CAD build for the part. Positions are in the model's coordinates, mm. A direction names the side the tool comes from. Give positions to 0.01 mm unless a question says otherwise; leave off trailing zeros. Loops run counter-clockwise (first coordinate to the right, second up) from the corner with the lowest first, then second, coordinate; pieces in that order, holes last. Notation, with made-up numbers: M 38.25,63.25 L 52.25,63.25 A29 cw 52.25,99.25 Z; hole C -14.5,-27 d10. An arc over 180 degrees is marked long. One line per question, with ' | ' between items.
```python
from build123d import *

# Parameters (mm, degrees)
BOSS_EXTRUDE1_DEPTH = 2
SKETCH2_R           = 3
SKETCH2_R_2         = 3.5
BOSS_EXTRUDE2_DEPTH = 3
SKETCH3_R           = 1.6
SKETCH3_R_2         = 2.1
CUT_EXTRUDE1_DEPTH  = 6


with BuildPart() as part:
    # Sketch1 → Boss-Extrude1 (new body)
    with BuildSketch(Plane.XY):
        with BuildLine():
            Line((0, 3), (6, 3))
            ThreePointArc((6, 3), (8.121320344, 3.878679656), (9, 6))
            Line((9, 6), (9, 12.5))
            ThreePointArc((9, 12.5), (9.878679656, 14.621320344), (12, 15.5))
            Line((12, 15.5), (21.823666576, 15.995555253))
            ThreePointArc((21.823666576, 15.995555253), (24.411724799, 15.036450964), (25.5, 12.5))
            Line((25.5, 12.5), (25.5, -7.5))
            ThreePointArc((25.5, -7.5), (23.339392013, -10.733578364), (19.525126266, -9.974873734))
            Line((19.525126266, -9.974873734), (12.550252532, -3))
            Line((12.550252532, -3), (0, -3))
            ThreePointArc((0, -3), (-3, 0), (0, 3))
        make_face()
    extrude(amount=BOSS_EXTRUDE1_DEPTH)

    # Sketch2 → Boss-Extrude2 (add)
    with BuildSketch(Plane.XY.offset(2)):
        Circle(SKETCH2_R)
        with Locations((12, 12.5)):
            Circle(SKETCH2_R)
        with Locations((22, 12.5)):
            Circle(SKETCH2_R_2)
        with Locations((22, -7.5)):
            Circle(SKETCH2_R_2)
    extrude(amount=BOSS_EXTRUDE2_DEPTH)

    # Sketch3 → Cut-Extrude1 (cut, through all)
    with BuildSketch(Plane.XY.offset(5)):
        Circle(SKETCH3_R)
        with Locations((12, 12.5)):
            Circle(SKETCH3_R)
        with Locations((22, 12.5)):
            Circle(SKETCH3_R_2)
        with Locations((22, -7.5)):
            Circle(SKETCH3_R_2)
    extrude(amount=-CUT_EXTRUDE1_DEPTH, mode=Mode.SUBTRACT)


solid = part.part
```
Item 1: Saw through at B-B on y = 0. Give the cut face in (x, z).
Conclusion:
outline: M -3,0 L -1.6,0 L -1.6,5 L -3,5 Z; M 1.6,0 L 25.5,0 L 25.5,2 L 3,2 L 3,5 L 1.6,5 Z
Item 2: Saw through at A-A on z = 3.8. Give the cut face in (x, y).
Conclusion:
outline: C 0,0 d6; C 12,12.5 d6; C 22,-7.5 d7; C 22,12.5 d7; hole C 0,0 d3.2; hole C 12,12.5 d3.2; hole C 22,-7.5 d4.2; hole C 22,12.5 d4.2
Item 3: 3-axis set-ups, long thin cutter, end or side, ignore diameter. For faces 1 (the flat face through (3, 3, 1)), 2 (the cylindrical face through (24.003, 13.131, 2.535)), 3 (the flat face through (16, 3, 2)), 4 (the flat face through (24, 11, 5)), 5 (the flat face through (6, -3, 1)): which of +Z, -Z, +X, -X, +Y, -Y reach the whole face in a straight line?
Conclusion:
face 1: +Z, -Z, -X, +Y | face 2: +Z, -Z | face 3: +Z | face 4: +Z, +X, -X, +Y, -Y | face 5: +Z, -Z, -X, -Y
Item 4: Mould opens along X. For faces 6 (the flat face through (9, 9, 1)), 7 (the flat face through (13, 11, 5)), 8 (the flat face through (25.5, 3, 1)), 9 (the cylindrical face through (10.4, 12.57, 2.54)) say: pulls with the +X half, pulls with the -X half, needs draft (parallel to the pull), parting line crosses it, or undercut.
Conclusion:
face 6: pulls with the -X half | face 7: needs draft | face 8: pulls with the +X half | face 9: undercut
Item 5: Drop flat-ended pins along their axis: P1, Ø8, axis at x = 12.5, y = 8.5, coming from the +Z side; P2, Ø1, axis at y = 2.5, z = 3.5, coming from the -X side; P3, Ø1, axis at y = 10, z = 0.5, coming from the -X side; P4, Ø0.6, axis at x = 2.5, z = 1, coming from the +Y side. Give the stop position or say it passes through.
Conclusion:
P1: z = 5 | P2: x = -2.24 | P3: x = 9 | P4: y = 3
Item 6: Drill centre lines: line 1 along Y through (x, z) = (22, 2.75); line 2 along Y through (x, z) = (12, 3.15); line 3 along Y through (x, z) = (22, 1.55). Where is each one in solid material? Low to high. Write a range as [from, to].
Conclusion:
line 1: [-11, -9.6], [-5.4, -4], [9, 10.4], [14.6, 16] | line 2: [9.5, 10.9], [14.1, 15.5] | line 3: [-11, -9.6], [-5.4, 10.4], [14.6, 16]
Item 7: Saw through at D-D on x = 1. Give the cut face in (y, z).
Conclusion:
outline: M -3,0 L -1.25,0 L -1.25,5 L -2.83,5 L -2.83,2 L -3,2 Z; M 1.25,0 L 3,0 L 3,2 L 2.83,2 L 2.83,5 L 1.25,5 Z
Item 8: Saw through at C-C on z = 0.5. Give the cut face in (x, y).
Conclusion:
outline: M 0,-3 L 12.55,-3 L 19.53,-9.97 A3.5 ccw 25.5,-7.5 L 25.5,12.5 A3.5 ccw 21.82,16 L 12,15.5 A3 ccw 9,12.5 L 9,6 A3 cw 6,3 L 0,3 A3 ccw Z; hole C 0,0 d3.2; hole C 12,12.5 d3.2; hole C 22,-7.5 d4.2; hole C 22,12.5 d4.2
